Check sheet for the drawn part. Datum: minimum x, y, z corner. Units: mm. Round coordinates to 2 decimals unless told otherwise and drop trailing zeros. Write each loop counter-clockwise with the first axis right and the second up, starting at its lowest first coordinate (ties: lowest second). Pieces come first, ordered by that corner, then holes. Notation, with made-up numbers: M 69.5,-8.75 L 105.5,-8.75 A30 cw 105.5,14.25 Z; hole C 18.5,60.5 d9. An arc over 180 degrees is marked long. One line per item, written item: value.
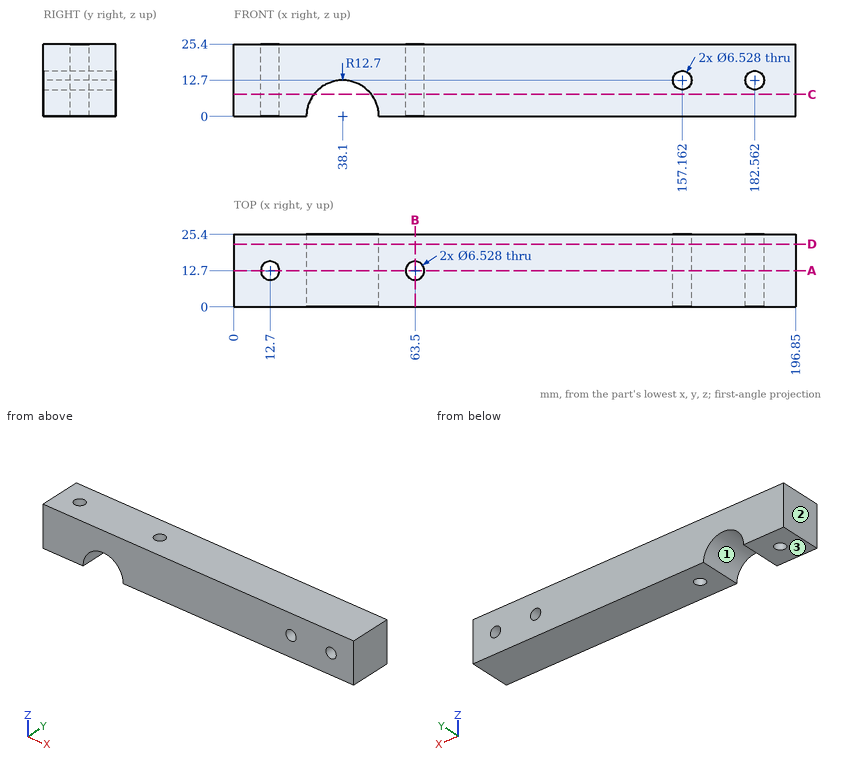
Q1. Sectioned sample at C-C on z = 7.75. Enter the section's corners in (x, y).
Completed:
outline: M 0,0 L 28.04,0 L 28.04,25.4 L 0,25.4 Z; M 48.16,0 L 196.85,0 L 196.85,25.4 L 48.16,25.4 Z; hole C 12.7,12.7 d6.53; hole C 63.5,12.7 d6.53
Q2. Sectioned sample at D-D on y = 22. Enter the section's corners in (x, z).
Completed:
outline: M 0,0 L 25.4,0 A12.7 cw 50.8,0 L 196.85,0 L 196.85,25.4 L 0,25.4 Z; hole C 157.16,12.7 d6.53; hole C 182.56,12.7 d6.53
Q3. Sectioned sample at B-B on x = 63.5. Enter the section's corners in (y, z), and give its area (3 significant figures).
Completed:
outline: M 0,0 L 9.44,0 L 9.44,25.4 L 0,25.4 Z; M 15.96,0 L 25.4,0 L 25.4,25.4 L 15.96,25.4 Z
area: 479 mm^2
Q4. Draft check along X on the marked faces 1, 2 and 3. Enter one of: pulls with the +X half, pulls with the -X half, needs draft (parallel to the pull), parting line crosses it, or undercut.
Completed:
face 1: undercut
face 2: pulls with the -X half
face 3: needs draft
Q5. Scan lines: line 1 (X direction, y = 12.5, z = 22.5); line 2 (Y direction, x = 63, z = 24) (1 decimal); line 3 (Y direction, x = 63.5, z = 12.5). Record each from-to range of solid material in increasing order. Write a range as [from, to].
Completed:
line 1: [0, 9.44], [15.96, 60.24], [66.76, 196.85]
line 2: [0, 9.5], [15.9, 25.4]
line 3: [0, 9.44], [15.96, 25.4]
Q6. Sectioned sample at A-A on y = 12.7. Enter the section's corners in (x, z).
Completed:
outline: M 0,0 L 9.44,0 L 9.44,25.4 L 0,25.4 Z; M 15.96,0 L 25.4,0 A12.7 cw 50.8,0 L 60.24,0 L 60.24,25.4 L 15.96,25.4 Z; M 66.76,0 L 196.85,0 L 196.85,25.4 L 66.76,25.4 Z; hole C 157.16,12.7 d6.53; hole C 182.56,12.7 d6.53
